Source: CAD feature listing. Evaluate the final solid. Frame: model axes, mm. Face numbers are marked on the shaded views. A direction names the side the tool comes from. Give positions to 0.01 mm unless a question says otherwise; leave off trailing zeros. Order: outer loops, then holes, each group sorted by start corner. A loop starts at its lowest first (then second) coordinate and runs counter-clockwise, first axis right, second up. Notation, with made-up numbers: (-16, 21.25) -> (43, 21.25) arc R16 cw to (43, 26.25) -> close; hole circle Ø11 at (80, -9.75). An arc over 180 degrees is marked (long way). Use CSV: the item, a comma, the result in double quotes.
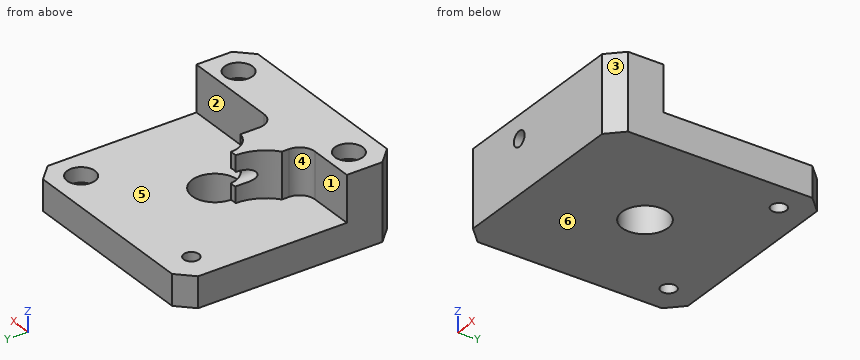
```python
from build123d import *

# Parameters (mm, degrees)
SKETCH_R        = 1.5
PAD_DEPTH       = 9
FILLET_R        = 3
SKETCH001_W     = 42.3
SKETCH001_H     = 42.3
SKETCH001_R     = 1.5
SKETCH001_R_2   = 4.5
PAD001_DEPTH    = 6
SKETCH002_R     = 1.5
POCKET_DEPTH    = 21.15
CHAMFER_SIZE    = 3
SKETCH003_R     = 2.75
POCKET001_DEPTH = 2.9
SKETCH004_R     = 2.75
POCKET002_DEPTH = 2.9


with BuildPart() as part:
    # Sketch → Pad (new body)
    with BuildSketch(Plane.XY):
        with BuildLine():
            Line((-21.15, -11.15), (-9.15, -11.15))
            Line((-9.15, -6.762211), (-9.15, -11.15))
            ThreePointArc((-9.15, -6.762211), (-6.683406, -3.773261), (-5.8, 0))
            Line((-5.8, 0), (-4.5, 0))
            ThreePointArc((-4.5, 0), (-3.46951, -2.865746), (-0.85, -4.418993))
            Line((-0.85, -4.418993), (-0.85, -11.15))
            Line((-0.85, -11.15), (21.15, -11.15))
            Line((21.15, -11.15), (21.15, -21.15))
            Line((21.15, -21.15), (-21.15, -21.15))
            Line((-21.15, -21.15), (-21.15, -11.15))
        make_face()
        with Locations((-15.5, -15.5)):
            Circle(SKETCH_R, mode=Mode.SUBTRACT)
        with Locations((15.5, -15.5)):
            Circle(SKETCH_R, mode=Mode.SUBTRACT)
    extrude(amount=PAD_DEPTH)

    # Fillet
    fillet_edges = [part.edges().sort_by_distance(p)[0] for p in [
        (-9.15, -11.15, 4.5),
        (-0.85, -11.15, 4.5),
    ]]
    fillet(fillet_edges, radius=FILLET_R)

    # Sketch001 → Pad001 (new body)
    with BuildSketch(Plane(origin=(0, 0, 0), x_dir=(1, 0, 0), z_dir=(0, 0, -1))):
        Rectangle(SKETCH001_W, SKETCH001_H)
        with Locations((15.5, -15.5)):
            Circle(SKETCH001_R, mode=Mode.SUBTRACT)
        with Locations((-15.5, -15.5)):
            Circle(SKETCH001_R, mode=Mode.SUBTRACT)
        Circle(SKETCH001_R_2, mode=Mode.SUBTRACT)
    extrude(amount=PAD001_DEPTH)

    # Sketch002 → Pocket (cut)
    with BuildSketch(Plane(origin=(0, 0, 0), x_dir=(-1, 0, 0), z_dir=(0, 1, 0))):
        with Locations((5.15, 4.5)):
            Circle(SKETCH002_R)
    extrude(amount=-POCKET_DEPTH, mode=Mode.SUBTRACT)

    # Chamfer
    chamfer_edges = [part.edges().sort_by_distance(p)[0] for p in [
        (-21.15, 21.15, -3),
        (-21.15, -21.15, -3),
        (21.15, -21.15, -3),
        (21.15, 21.15, -3),
    ]]
    chamfer(chamfer_edges, length=CHAMFER_SIZE)

    # Sketch003 → Pocket001 (cut)
    with BuildSketch(Plane.XY.offset(9)):
        with Locations((15.5, -15.5)):
            Circle(SKETCH003_R)
        with Locations((-15.5, -15.5)):
            Circle(SKETCH003_R)
    extrude(amount=-POCKET001_DEPTH, mode=Mode.SUBTRACT)

    # Sketch004 → Pocket002 (cut)
    with BuildSketch(Plane.XY):
        with Locations((15.5, 15.5)):
            Circle(SKETCH004_R)
    extrude(amount=-POCKET002_DEPTH, mode=Mode.SUBTRACT)


solid = part.part
```
1. Section query B-B on z = 1.25. Return loops of the section in (x, y), plus the area to 3 significant figures.
Answer below:
outline,"(-21.15, -18.15) -> (-18.15, -21.15) -> (18.15, -21.15) -> (21.15, -18.15) -> (21.15, -11.15) -> (2.15, -11.15) arc R3 cw to (-0.85, -8.15) -> (-0.85, -4.42) arc R4.5 cw to (-4.5, 0) -> (-5.8, 0) arc R8.5 cw to (-9.15, -6.76) -> (-9.15, -8.15) arc R3 cw to (-12.15, -11.15) -> (-21.15, -11.15) -> close; hole circle Ø3 at (-15.5, -15.5); hole circle Ø3 at (15.5, -15.5)"
area,"468 mm²"
2. Section query C-C on z = 5.25. Return loops of the section in (x, y), plus the area to 3 significant figures.
Answer below:
outline,"(-21.15, -18.15) -> (-18.15, -21.15) -> (-6.45, -21.15) -> (-6.45, -3.26) arc R8.5 cw to (-9.15, -6.76) -> (-9.15, -8.15) arc R3 cw to (-12.15, -11.15) -> (-21.15, -11.15) -> close; (-3.85, -21.15) -> (18.15, -21.15) -> (21.15, -18.15) -> (21.15, -11.15) -> (2.15, -11.15) arc R3 cw to (-0.85, -8.15) -> (-0.85, -4.42) arc R4.5 cw to (-3.85, -2.33) -> close; hole circle Ø3 at (-15.5, -15.5); hole circle Ø3 at (15.5, -15.5)"
area,"416 mm²"
3. Section query A-A on x = 15.5. Return loops of the section in (y, z), plus the area to 3 significant figures.
Answer below:
outline,"(-21.15, -6) -> (14, -6) -> (14, -2.9) -> (12.75, -2.9) -> (12.75, 0) -> (-11.15, 0) -> (-11.15, 9) -> (-12.75, 9) -> (-12.75, 6.1) -> (-14, 6.1) -> (-14, 0) -> (-17, 0) -> (-17, 6.1) -> (-18.25, 6.1) -> (-18.25, 9) -> (-21.15, 9) -> close; (17, -6) -> (21.15, -6) -> (21.15, 0) -> (18.25, 0) -> (18.25, -2.9) -> (17, -2.9) -> close"
area,"284 mm²"
4. Section query D-D on y = -15.5. Return loops of the section in (x, z), plus the area to 3 significant figures.
Answer below:
outline,"(-21.15, -6) -> (21.15, -6) -> (21.15, 9) -> (18.25, 9) -> (18.25, 6.1) -> (17, 6.1) -> (17, 0) -> (14, 0) -> (14, 6.1) -> (12.75, 6.1) -> (12.75, 9) -> (-12.75, 9) -> (-12.75, 6.1) -> (-14, 6.1) -> (-14, 0) -> (-17, 0) -> (-17, 6.1) -> (-18.25, 6.1) -> (-18.25, 9) -> (-21.15, 9) -> close; hole circle Ø3 at (-5.15, 4.5)"
area,"559 mm²"
5. Pin query (flat end, axial travel): P1, Ø6, axis at x = 15.5, y = -16.5, coming from the +Z side; P2, Ø7, axis at x = 11, z = 6.5, coming from the +Y side; P3, Ø2.5, axis at x = 15.5, y = -15.5, coming from the +Z side; P4, Ø3, axis at y = -6, z = 4.5, coming from the +X side. Return the tip coordinate at first contact, or that it passes through.
Answer below:
P1,"stops at z = 9"
P2,"stops at y = -11.15"
P3,"stops at z = 0"
P4,"stops at x = -0.85"
6. Access query for the marked faces 1, 2 and 3. Directions: +Z, -Z, +X, -X, +Y, -Y. A direction counts if a zero-diameter tool reaches every point of the face in a straight line with its end or side. Return the directions, or none.
Answer below:
face 1,"+Z, -X, +Y"
face 2,"+Z, +X, +Y"
face 3,"+Z, -Z, +X, -Y"
7. Ray query, line 1 along X through (y, z) = (-15.5, 1.5); line 2 along Y through (x, z) = (15.5, -0.8); line 3 along Y through (x, z) = (0, -0.5). Return the intervals inside material, ascending.
Answer below:
line 1,"x = -21.15 to -17, -14 to 14, 17 to 21.15"
line 2,"y = -21.15 to 12.75, 18.25 to 21.15"
line 3,"y = -21.15 to -4.5, 4.5 to 21.15"
8. Mould query, pull axis Z, two halves, no side actions, for the marked faces 4, 5 and 6. Classes: released by +Z, released by -Z, zero draft, split by the parting line, or undercut.
Answer below:
face 4,"zero draft"
face 5,"released by +Z"
face 6,"released by -Z"
